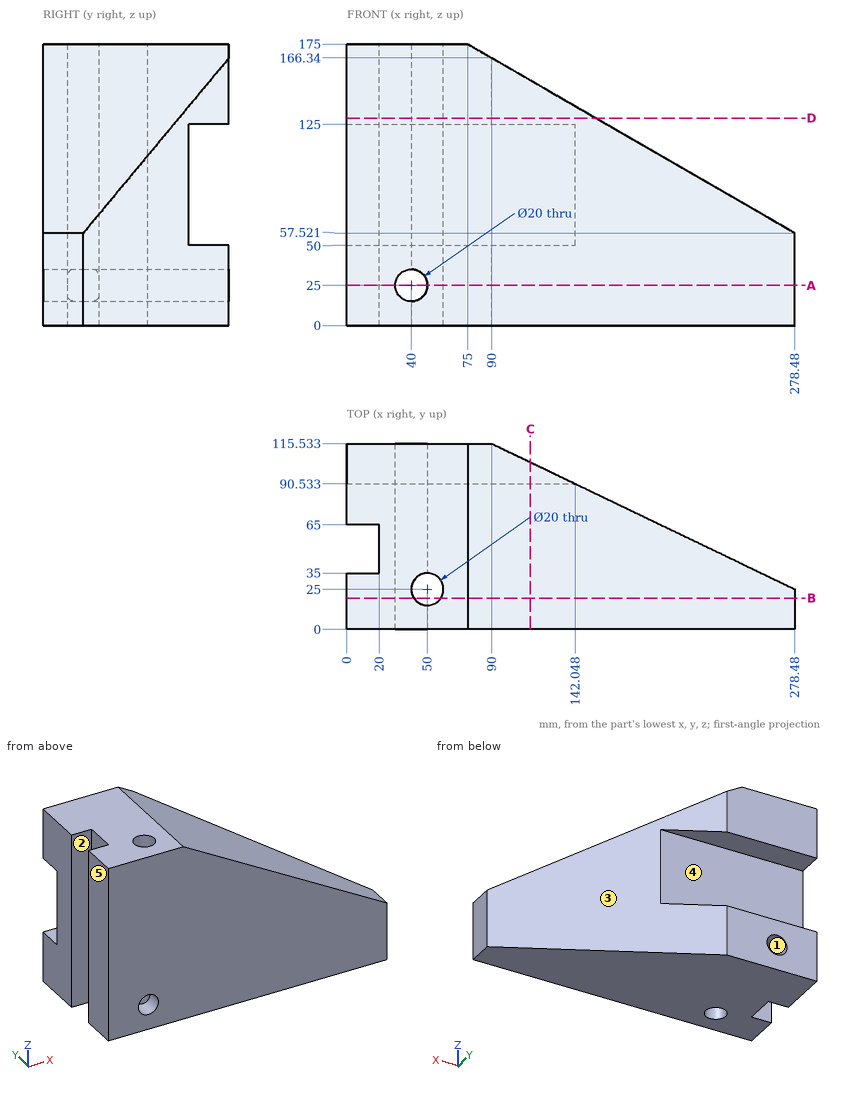
Study the drawing (mm; zero at the part's minimum x, y, z) and answer. A direction names the side the tool comes from. Give positions to 0.01 mm unless a question says otherwise; leave off trailing zeros. Loops run counter-clockwise (first coordinate to the right, second up) from the corner with the lowest first, then second, coordinate; pieces in that order, holes last. Notation, with made-up numbers: (-3.5, -3.75) - (18.5, -3.75) arc R27 cw to (18.5, 33.25) - close; hole circle Ø11 at (88, -7.5). An arc over 180 degrees is marked (long way). Return JSON: item names as keys, results as strings. Group by question number.
1. Which of the six approach directions +Z, -Z, +X, -X, +Y, -Y give full straight-line access (tool end or side, diameter ignored) to the marked faces 4 and 5?
2. Find section A-A (z = 25). Write down the section's boundary in (x, y), then the cut area to 3 significant figures.
3. Given pin 1 Ø15 at (y, z) = (52, 131) entering from -X; pin 2 Ø1.5 at (y, z) = (76.5, 121.5) entering from +X (1 decimal); pin 3 Ø6 at (x, y) = (195.5, 68) entering from +Z, each flat-ended and moving along its own axis, determine where each tip first touches the part or whether it passes through.
4. Find section D-D (z = 129). Write down the section's boundary in (x, y) (1 decimal), then the cut area to 3 significant figures.
5. Straight lines are drawn through the part: line 1 (Z direction, x = 60, y = 97.5); line 2 (Y direction, x = 50, z = 82); line 3 (Z direction, x = 40, y = 62). For each, find the intervals that lie inside material, in ascending order. Write a range as [from, to].
6. Find section B-B (y = 19.5). Write down the section's boundary in (x, z), then the cut area to 3 significant figures.
7. Find section C-C (x = 114). Write down the section's boundary in (y, z) (1 decimal).
8. Determine the mould class of the marked faces 1, 2 and 3 for opening direction Y: pulls with the +Y half, pulls with the -Y half, needs draft (parallel to the pull), parting line crosses it, or undercut.
Verdict:
{
 "1": {"face 4": "+X, -X, +Y", "face 5": "+Z, -Z, -X, +Y, -Y"},
 "2": {"outline": "(0, 0) - (30, 0) - (30, 115.53) - (0, 115.53) - (0, 65) - (20, 65) - (20, 35) - (0, 35) - close; (50, 0) - (278.48, 0) - (278.48, 25) - (90, 115.53) - (50, 115.53) - (50, 35) arc R10 cw to (50, 15) - close", "area": "20,600 mm^2"},
 "3": {"pin 1": "stops at x = 20", "pin 2": "stops at x = 169", "pin 3": "stops at z = 106.65"},
 "4": {"outline": "(0, 0) - (154.7, 0) - (154.7, 84.5) - (90, 115.5) - (0, 115.5) - (0, 65) - (20, 65) - (20, 35) - (0, 35) - close; hole circle Ø20 at (50, 25)", "area": "16,000 mm^2"},
 "5": {"line 1": "z = [0, 50], [125, 175]", "line 2": "y = [0, 15], [35, 90.53]", "line 3": "z = [0, 15], [35, 175]"},
 "6": {"outline": "(0, 0) - (41.65, 0) - (41.65, 15.14) arc R10 cw (long way) to (41.65, 34.86) - (41.65, 175) - (0, 175) - close; (58.35, 0) - (278.48, 0) - (278.48, 57.52) - (75, 175) - (58.35, 175) - close", "area": "33,700 mm^2"},
 "7": {"outline": "(0, 0) - (104, 0) - (104, 50) - (90.5, 50) - (90.5, 125) - (104, 125) - (104, 152.5) - (0, 152.5) - close"},
 "8": {"face 1": "needs draft", "face 2": "undercut", "face 3": "pulls with the +Y half"}
}
